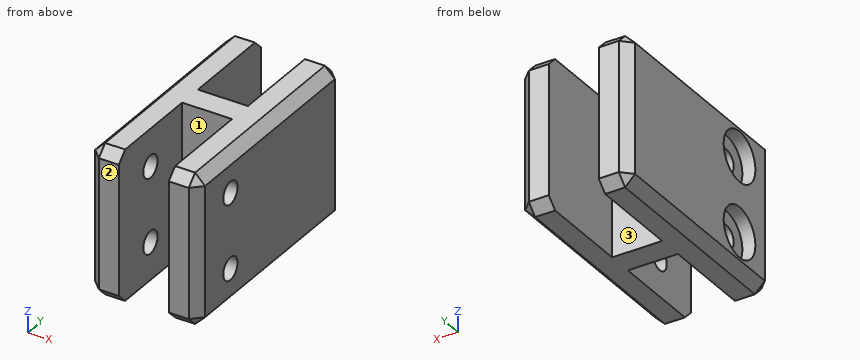
```python
from build123d import *

# Parameters (mm, degrees)
ESTRUSIONE_ESTRUSIONE1_DEPTH                         = 30
FORO_LAMATO_PER_VITE_M4_A_TESTA_CILINDRI_D           = 4.5
FORO_LAMATO_PER_VITE_M4_A_TESTA_CILINDRI_DEPTH       = 30
FORO_LAMATO_PER_VITE_M4_A_TESTA_CILINDRI_CBORE_D     = 10
FORO_LAMATO_PER_VITE_M4_A_TESTA_CILINDRI_CBORE_DEPTH = 2.6
FORO_LAMATO_PER_VITE_M4_A_TESTA_CILINDRI_TIP         = 1.351936393
SMUSSO1_SIZE                                         = 2


with BuildPart() as part:
    # Schizzo1 → Estrusione-Estrusione1 (new body)
    with BuildSketch(Plane.XY):
        Polygon((11, -25), (11, 20), (5, 20), (5, 0), (-5, 0), (-5, 20), (-11, 20), (-11, -25), (-5, -25), (-5, -5), (5, -5), (5, -25), align=None)
    extrude(amount=ESTRUSIONE_ESTRUSIONE1_DEPTH)

    # Foro lamato per Vite M4 a testa cilindrica piana-1
    with Locations(Plane(origin=(-11, -15, 22.5), x_dir=(0, -1, 0), z_dir=(-1, 0, 0))):
        with Locations((0, 0), (0, -15)):
            CounterBoreHole(FORO_LAMATO_PER_VITE_M4_A_TESTA_CILINDRI_D / 2, FORO_LAMATO_PER_VITE_M4_A_TESTA_CILINDRI_CBORE_D / 2, FORO_LAMATO_PER_VITE_M4_A_TESTA_CILINDRI_CBORE_DEPTH, depth=FORO_LAMATO_PER_VITE_M4_A_TESTA_CILINDRI_DEPTH)
            with Locations((0, 0, -(FORO_LAMATO_PER_VITE_M4_A_TESTA_CILINDRI_DEPTH + FORO_LAMATO_PER_VITE_M4_A_TESTA_CILINDRI_TIP / 2))):  # 118° drill point
                Cone(0, FORO_LAMATO_PER_VITE_M4_A_TESTA_CILINDRI_D / 2, FORO_LAMATO_PER_VITE_M4_A_TESTA_CILINDRI_TIP, mode=Mode.SUBTRACT)

    # Smusso1
    smusso1_edges = [part.edges().sort_by_distance(p)[0] for p in [
        (-8, -25, 30),
        (8, 20, 0),
        (11, -2.5, 0),
        (8, -25, 0),
        (-8, -25, 0),
        (-11, -2.5, 0),
        (-8, 20, 0),
        (11, 20, 15),
        (11, -25, 15),
        (-11, -25, 15),
        (-11, 20, 15),
        (8, -25, 30),
        (11, -2.5, 30),
        (8, 20, 30),
        (-8, 20, 30),
        (-11, -2.5, 30),
    ]]
    chamfer(smusso1_edges, length=SMUSSO1_SIZE)


solid = part.part
```
Could you check a few things on this model? Use its own coordinates, in mm. Face numbers are marked on the shaded views. A direction names the side the tool comes from. Coordinates: 2 decimals unless noted, no trailing zeros. Loops run counter-clockwise (first coordinate to the right, second up) from the corner with the lowest first, then second, coordinate; pieces in that order, holes last.
1) Imagine slicing it at C-C (z = 22.5). List the corners of the cut face in (x, y) for me, and give its area (3 significant figures).
Reported:
outline: (-11, -23) - (-9, -25) - (-5, -25) - (-5, -17.25) - (-8.4, -17.25) - (-8.4, -20) - (-11, -20) - close; (-11, -10) - (-8.4, -10) - (-8.4, -12.75) - (-5, -12.75) - (-5, -5) - (5, -5) - (5, -12.75) - (11, -12.75) - (11, 18) - (9, 20) - (5, 20) - (5, 0) - (-5, 0) - (-5, 20) - (-9, 20) - (-11, 18) - close; (5, -25) - (9, -25) - (11, -23) - (11, -17.25) - (5, -17.25) - close
area: 514 mm2
2) Imagine slicing it at B-B (x = 9.5). List the corners of the cut face in (y, z) for me.
Reported:
outline: (-24.5, 2) - (-23, 0.5) - (18, 0.5) - (19.5, 2) - (19.5, 28) - (18, 29.5) - (-23, 29.5) - (-24.5, 28) - close; hole circle Ø4.5 at (-15, 7.5); hole circle Ø4.5 at (-15, 22.5)
3) Will these pins go through, and if not, where does the flat tip stop? pin 1 Ø3.5 at (y, z) = (-15, 22.5) entering from -X; pin 2 Ø3 at (x, z) = (2.5, 22) entering from -Y; pin 3 Ø3 at (x, z) = (0.5, 21) entering from +Y.
Reported:
pin 1: passes through
pin 2: stops at y = -5
pin 3: stops at y = 0
4) Which directions (+Z, -Z, +X, -X, +Y, -Y) give clear straight access to the entire face, cutting with the end or side of a thin tool? Please do the marked faces 1, 2 and 3.
Reported:
face 1: +Z, -Z, -Y
face 2: +Z, -Z, +X, -X, -Y
face 3: +Z, -Z, +Y
5) Imagine slicing it at D-D (z = 15). List the corners of the cut face in (x, y) for me.
Reported:
outline: (-11, -23) - (-9, -25) - (-5, -25) - (-5, -5) - (5, -5) - (5, -25) - (9, -25) - (11, -23) - (11, 18) - (9, 20) - (5, 20) - (5, 0) - (-5, 0) - (-5, 20) - (-9, 20) - (-11, 18) - close
6) Imagine slicing it at A-A (y = 8.5). List the corners of the cut face in (x, z) for me, and give its area (3 significant figures).
Reported:
outline: (-11, 2) - (-9, 0) - (-5, 0) - (-5, 30) - (-9, 30) - (-11, 28) - close; (5, 0) - (9, 0) - (11, 2) - (11, 28) - (9, 30) - (5, 30) - close
area: 352 mm2
7) Please list where these lines run through material, in increasing order: line 1 along Z through (x, y) = (6.85, -15); line 2 along Z through (x, y) = (-8.95, -15); line 3 along X through (y, z) = (17, 17.5).
Reported:
line 1: z = 0 to 5.25, 9.75 to 20.25, 24.75 to 30
line 2: z = 0 to 2.5, 12.5 to 17.5, 27.5 to 30
line 3: x = -11 to -5, 5 to 11
